from build123d import *

# Parameters (mm, degrees)
F0_W     = 7.5
F0_H     = 41
F1_DEPTH = 20
F2_DEPTH = 10
F3_SIZE  = 9.99999
F4_W     = 10
F4_H     = 10
F5_DEPTH = 195.501
F7_DEPTH = 10
F8_R     = 0.75
F9_DEPTH = 25


# Not quite as in the source:
# - a fillet or chamfer is up to 0.001 mm smaller than in the source, because OpenCascade refuses the exact size


with BuildPart() as f1:
    # F0 (on Top) → F1 (new body)
    with BuildSketch(Plane.XY):
        Polygon((-12.5, 80), (-12.5, 75), (-12.5, -115.5), (5, -115.5), (5, -110.5), (5, 80), align=None)
        Polygon((0, 34), (0, 0), (0, -7.5), (0, -69.5), (0, -110.5), (-7.5, -110.5), (-7.5, -69.5), (-7.5, 34), (-7.5, 75), (0, 75), align=None, mode=Mode.SUBTRACT)
        with Locations((-3.75, -90)):
            Rectangle(F0_W, F0_H)
        Polygon((0, -7.5), (0, 0), (0, 34), (-7.5, 34), (-7.5, -69.5), (0, -69.5), align=None)
        with Locations((-3.75, 54.5)):
            Rectangle(F0_W, F0_H)
    extrude(amount=-F1_DEPTH)

    # F0 (on Top) → F2 (cut)
    with BuildSketch(Plane.XY):
        with Locations((-3.75, 54.5)):
            Rectangle(F0_W, F0_H)
        with Locations((-3.75, -90)):
            Rectangle(F0_W, F0_H)
    extrude(amount=-F2_DEPTH, mode=Mode.SUBTRACT)

    # F3 (size 10 in the source; OpenCascade refuses exactly that, so slightly less here)
    f3_edges = [f1.edges().sort_by_distance(p)[0] for p in [
        (-3.75, -69.5, -10),
        (-3.75, 34, -10),
    ]]
    chamfer(f3_edges, length=F3_SIZE)

    # F4 (on face) → F5 (cut, through all)
    with BuildSketch(Plane.XZ.offset(115.5)):
        with Locations((0, -15)):
            Rectangle(F4_W, F4_H)
    extrude(amount=-F5_DEPTH, mode=Mode.SUBTRACT)

    # F6 (on face) → F7 (join)
    with BuildSketch(Plane.XY):
        with BuildLine():
            Line((29, -22.6551367564), (5, -3.9060580615))
            Line((5, -3.9060580615), (5, -54.0939419385))
            Line((5, -54.0939419385), (32.0781262822, -32.9401952478))
            ThreePointArc((32.0781262822, -32.9401952478), (26.8080409916, -33.4939198597), (24, -29))
            ThreePointArc((24, -29), (25.4644660941, -25.4644660941), (29, -24))
            Line((29, -24), (29, -22.6551367564))
        make_face()
        with BuildLine():
            Line((32.0781262822, -25.0598047522), (29, -22.6551367564))
            Line((29, -22.6551367564), (29, -24))
            ThreePointArc((29, -24), (30.627732128, -24.2723697142), (32.0781262822, -25.0598047522))
        make_face()
        with BuildLine():
            ThreePointArc((32.0781262822, -25.0598047522), (30.627732128, -24.2723697142), (29, -24))
            Line((29, -24), (29, -28.5))
            ThreePointArc((29, -28.5), (29.3535533906, -28.6464466094), (29.5, -29))
            ThreePointArc((29.5, -29), (29, -29.5), (28.5, -29))
            Line((28.5, -29), (24, -29))
            ThreePointArc((24, -29), (26.8080409916, -33.4939198597), (32.0781262822, -32.9401952478))
            ThreePointArc((32.0781262822, -32.9401952478), (33.4939198597, -31.1919590084), (34, -29))
            ThreePointArc((34, -29), (33.4939198597, -26.8080409916), (32.0781262822, -25.0598047522))
        make_face()
        with BuildLine():
            Line((29, -28.5), (29, -24))
            ThreePointArc((29, -24), (25.4644660941, -25.4644660941), (24, -29))
            Line((24, -29), (28.5, -29))
            ThreePointArc((28.5, -29), (28.6464466094, -28.6464466094), (29, -28.5))
        make_face()
    extrude(amount=-F7_DEPTH)

    # F8 (on face) → F9 (cut)
    with BuildSketch(Plane(origin=(0, 0, -10), x_dir=(1, 0, 0), z_dir=(0, 0, -1))):
        with Locations((23, 29)):
            Circle(F8_R)
        with BuildLine():
            ThreePointArc((26.537409976, 32.5336568398), (27.6199052956, 30.9121911672), (28, 29))
            ThreePointArc((28, 29), (27.6199052956, 27.0878088328), (26.537409976, 25.4663431602))
            Line((26.537409976, 25.4663431602), (5, 3.9060580615))
            Line((5, 3.9060580615), (32.0781262822, 25.0598047522))
            ThreePointArc((32.0781262822, 25.0598047522), (34, 29), (32.0781262822, 32.9401952478))
            Line((32.0781262822, 32.9401952478), (5, 54.0939419385))
            Line((5, 54.0939419385), (26.537409976, 32.5336568398))
        make_face()
        with BuildLine():
            ThreePointArc((29.5, 29), (29, 28.5), (28.5, 29))
            ThreePointArc((28.5, 29), (29, 29.5), (29.5, 29))
        make_face(mode=Mode.SUBTRACT)
    extrude(amount=-F9_DEPTH, mode=Mode.SUBTRACT)


solid = f1.part
Model file for the job. Use its own axes, mm. A direction names the side the tool comes from. Give positions to 0.01 mm unless a question says otherwise; leave off trailing zeros. Order: outer loops, then holes, each group sorted by start corner. A loop starts at its lowest first (then second) coordinate and runs counter-clockwise, first axis right, second up. Notation, with made-up numbers: M 69.25,5 L 125.25,5 A30 ccw 125.25,44 Z; hole C 5,34.25 d6. An arc over 180 degrees is marked long. Write item = value, one per line.
Q1. Cut at D-D, the plane x = 9. List the corners of the cut face in (y, z).
Derived:
outline = M -50.09,-10 L -7.91,-10 L -7.91,0 L -50.09,0 Z
Q2. Two-plate mould, pull along X, no slides. Class faces 1 (the flat face through (-7.5, -95, -5)), 2 (the flat face through (-5, -19, -15)), 3 (the flat face through (-6, -115.5, -8)): pulls with the +X half, pulls with the -X half, needs draft (parallel to the pull), parting line crosses it, or undercut.
Derived:
face_1 = undercut
face_2 = pulls with the +X half
face_3 = needs draft
Q3. Tool access for faces 4 (the flat face through (4, -19, -10)), 5 (the flat face through (5, -85, -5)), 6 (the flat face through (-12.5, -16, -10)), 7 (the flat face through (5, 37, -5)), 8 (the flat face through (-3.8, -74.6, -5.1)): list every direction of +Z, -Z, +X, -X, +Y, -Y with a clear straight run to the whole face (end or side of a thin tool).
Derived:
face_4 = -Z, +X, +Y, -Y
face_5 = +Z, -Z, +X, -Y
face_6 = +Z, -Z, -X, +Y, -Y
face_7 = +Z, -Z, +X, +Y
face_8 = +Z
Q4. Cut at A-A, the plane y = 49.5. List the corners of the cut face in (x, z), then the cut area to 3 significant figures.
Derived:
outline = M -12.5,-20 L -5,-20 L -5,-10 L -7.5,-10 L -7.5,0 L -12.5,0 Z; M 0,-10 L 5,-10 L 5,0 L 0,0 Z
area = 175 mm2
Q5. Drill centre lines: line 1 (X direction, y = -105.5, z = -5.5); line 2 (X direction, y = -29, z = -6.25); line 3 (X direction, y = -52, z = -11.25). Where is each one in solid material? Low to high. Write a range as [from, to].
Derived:
line_1 = [-12.5, -7.5], [0, 5]
line_2 = [-12.5, 22.25], [23.75, 28]
line_3 = [-12.5, -5]
Q6. Cut at B-B, the plane z = -12.5. List the corners of the cut face in (x, y), then the cut area to 3 significant figures.
Derived:
outline = M -12.5,-115.5 L -5,-115.5 L -5,80 L -12.5,80 Z
area = 1,470 mm2
Q7. Cut at C-C, the plane y = -7. List the corners of the cut face in (x, z).
Derived:
outline = M -12.5,-20 L -5,-20 L -5,-10 L 8.09,-10 L 8.09,0 L -12.5,0 Z
Q8. Flat gauge pins, fed straight in: pin 1 (2 mm diameter, centred on x = 23, y = -29, fed in from -Z); pin 2 (0.8 mm diameter, centred on x = -7, y = 54.5, fed in from +Z); pin 3 (3 mm diameter, centred on y = -0.5, z = -16.5, fed in from +X). Where does each tip first touch, or does it go through?
Derived:
pin_1 = -10
pin_2 = -10
pin_3 = -5
